Can you work these out from the model? Positions are in its coordinate system, mm. Face numbers are marked on the shaded views. A direction names the side the tool comes from. Round coordinates to 2 decimals unless told otherwise and drop trailing zeros. Order: outer loops, then holes, each group sorted by start corner. A loop starts at its lowest first (then second) coordinate and runs counter-clockwise, first axis right, second up.
Q1. If I drill on line 1 (Z direction, x = 0, y = 0); line 2 (Y direction, x = 3, z = 0); line 3 (Z direction, x = -12, y = 17.5), over which ranges is the centre line in solid material (lowest first)?
Q2. If we section it at D-D (z = 5.5): Please give me the cut outline in (x, y), plus the area to 3 significant figures.
Q3. If we section it at C-C (z = -5.5): Please give me the cut outline in (x, y).
Q4. We'd pull the mould along Y, two halves only. Please class the marked faces 1, 2, 3 and 4: pulls with the +Y half, pulls with the -Y half, needs draft (parallel to the pull), parting line crosses it, or undercut.
Q5. Will these pins go through, and if not, where does the flat tip stop? P1, Ø1.5, axis at y = 8.5, z = 10, coming from the +X side; P2, Ø3, axis at x = 2.5, z = -0.5, coming from the +Y side; P3, Ø12, axis at x = -16, z = -8, coming from the +Y side; P4, Ø6.5, axis at x = 1.5, z = -12, coming from the -Y side.
Q6. For the marked faces 5, 6, 7 and 8, which set-ups out of +Z, -Z, +X, -X, +Y, -Y let a thin tool reach every point of the face, with its end or its side?
Q7. If we section it at B-B (x = 0): Please give me the cut outline in (y, z).
Q8. If we section it at A-A (y = 0): Please give me the cut outline in (x, z), plus the area to 3 significant figures.
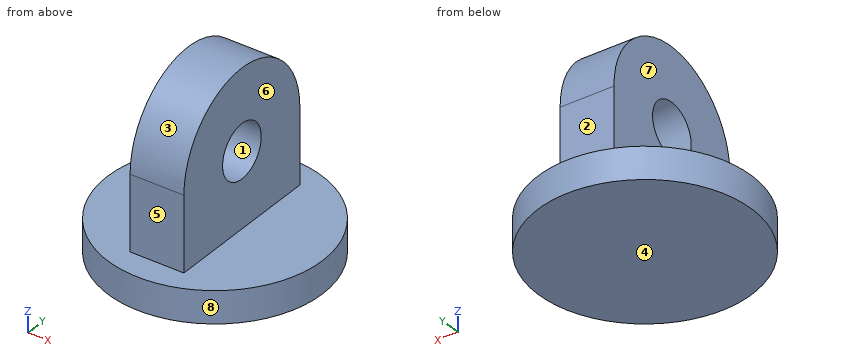
from build123d import *

# Parameters (mm, degrees)
F0_R     = 25.4
F1_DEPTH = 25.4
F2_W     = 25.4
F2_H     = 76.2
F2_H_2   = 76.310582
F3_DEPTH = 43.18
F4_R     = 6.35
F4_W     = 19.05
F4_H     = 17.78
F5_DEPTH = 25.4


with BuildPart() as f1:
    # F0 (on Top) → F1 (new body, symmetric)
    with BuildSketch(Plane.XY):
        Circle(F0_R)
    extrude(amount=F1_DEPTH, both=True)

    # F2 (on face) → F3 (cut)
    with BuildSketch(Plane.XY.offset(25.4)):
        with Locations((-19.05, 0)):
            Rectangle(F2_W, F2_H)
        with Locations((19.05, -0.055291)):
            Rectangle(F2_W, F2_H_2)
    extrude(amount=-F3_DEPTH, mode=Mode.SUBTRACT)

    # F4 (on Right) → F5 (cut, symmetric)
    with BuildSketch(Plane.YZ):
        Circle(F4_R)
        with BuildLine():
            ThreePointArc((-19.05, 0), (0, 19.05), (19.05, 0))
            Line((19.05, 0), (38.1, 0))
            Line((38.1, 0), (38.1, 38.1))
            Line((38.1, 38.1), (-38.1, 38.1))
            Line((-38.1, 38.1), (-38.1, 0))
            Line((-38.1, 0), (-19.05, 0))
        make_face()
        with Locations((28.575, -8.89)):
            Rectangle(F4_W, F4_H)
        with Locations((-28.575, -8.89)):
            Rectangle(F4_W, F4_H)
    extrude(amount=F5_DEPTH, both=True, mode=Mode.SUBTRACT)


solid = f1.part
Solution:
1. line 1: z = -25.4 to -6.35, 6.35 to 19.05
1. line 2: y = -19.05 to -6.35, 6.35 to 19.05
1. line 3: z = -25.4 to -17.78
2. outline: (-6.35, -18.24) - (6.35, -18.24) - (6.35, -3.17) - (-6.35, -3.17) - close; (-6.35, 3.17) - (6.35, 3.17) - (6.35, 18.24) - (-6.35, 18.24) - close
2. area: 383 mm2
3. outline: (-6.35, -19.05) - (6.35, -19.05) - (6.35, -3.17) - (-6.35, -3.17) - close; (-6.35, 3.17) - (6.35, 3.17) - (6.35, 19.05) - (-6.35, 19.05) - close
4. face 1: undercut
4. face 2: pulls with the +Y half
4. face 3: parting line crosses it
4. face 4: needs draft
5. P1: stops at x = 6.35
5. P2: stops at y = 19.05
5. P3: passes through
5. P4: stops at y = -19.05
6. face 5: +Z, +X, -X, -Y
6. face 6: +Z, +X, +Y, -Y
6. face 7: +Z, -X, +Y, -Y
6. face 8: +Z, -Z
7. outline: (-25.4, -25.4) - (25.4, -25.4) - (25.4, -17.78) - (19.05, -17.78) - (19.05, 0) arc R19.05 ccw to (-19.05, 0) - (-19.05, -17.78) - (-25.4, -17.78) - close; hole circle Ø12.7 at (0, 0)
8. outline: (-25.4, -25.4) - (25.4, -25.4) - (25.4, -17.78) - (6.35, -17.78) - (6.35, -6.35) - (-6.35, -6.35) - (-6.35, -17.78) - (-25.4, -17.78) - close; (-6.35, 6.35) - (6.35, 6.35) - (6.35, 19.05) - (-6.35, 19.05) - close
8. area: 694 mm2
